from build123d import *

# Parameters (mm, degrees)
F0_R      = 19.05
F1_DEPTH  = 15.875
F2_R      = 9.525
F3_DEPTH  = 12.7
F5_R      = 1.5875
F6_DEPTH  = 25.4
F7_R      = 1.582292
F8_DEPTH  = 25.4
F9_R      = 1.5875
F10_DEPTH = 25.4
F11_R     = 1.5875
F12_DEPTH = 25.4
F13_R     = 1.5875
F14_DEPTH = 25.4
F15_R     = 1.5875
F16_DEPTH = 25.4
F17_R     = 1.5875
F18_DEPTH = 25.4
F19_R     = 1.5875
F20_DEPTH = 25.4
F21_R     = 4.7625
F22_DEPTH = 1.5875
F23_R     = 2.38125
F24_DEPTH = 1.5875
F26_R     = 18.052575
F26_R_2   = 9.68479
F27_DEPTH = 13.462
F28_R     = 3.175
F29_DEPTH = 9.652
F30_R     = 1.5875
F31_DEPTH = 10.668


with BuildPart() as f1:
    # F0 (on Front) → F1 (new body)
    with BuildSketch(Plane.XZ):
        Circle(F0_R)
    extrude(amount=-F1_DEPTH)

    # F2 (on face) → F3 (cut)
    with BuildSketch(Plane.XZ):
        Circle(F2_R)
    extrude(amount=-F3_DEPTH, mode=Mode.SUBTRACT)

    # F5 (on face) → F6 (cut)
    with BuildSketch(Plane.XZ.offset(-12.7)):
        with Locations((0, 7.420709)):
            Circle(F5_R)
    extrude(amount=-F6_DEPTH, mode=Mode.SUBTRACT)

    # F7 (on face) → F8 (cut)
    with BuildSketch(Plane.XZ.offset(-12.7)):
        with Locations((0, -7.351812)):
            Circle(F7_R)
    extrude(amount=-F8_DEPTH, mode=Mode.SUBTRACT)

    # F9 (on face) → F10 (cut)
    with BuildSketch(Plane.XZ.offset(-12.7)):
        with Locations((-7.360636, 0)):
            Circle(F9_R)
    extrude(amount=-F10_DEPTH, mode=Mode.SUBTRACT)

    # F11 (on face) → F12 (cut)
    with BuildSketch(Plane.XZ.offset(-12.7)):
        with Locations((7.366985, 0)):
            Circle(F11_R)
    extrude(amount=-F12_DEPTH, mode=Mode.SUBTRACT)

    # F13 (on face) → F14 (cut)
    with BuildSketch(Plane.XZ.offset(-12.7)):
        with Locations((-5.115572, 5.085843)):
            Circle(F13_R)
    extrude(amount=-F14_DEPTH, mode=Mode.SUBTRACT)

    # F15 (on face) → F16 (cut)
    with BuildSketch(Plane.XZ.offset(-12.7)):
        with Locations((5.301525, 5.085843)):
            Circle(F15_R)
    extrude(amount=-F16_DEPTH, mode=Mode.SUBTRACT)

    # F17 (on face) → F18 (cut)
    with BuildSketch(Plane.XZ.offset(-12.7)):
        with Locations((-5.205374, -5.196551)):
            Circle(F17_R)
    extrude(amount=-F18_DEPTH, mode=Mode.SUBTRACT)

    # F19 (on face) → F20 (cut)
    with BuildSketch(Plane.XZ.offset(-12.7)):
        with Locations((5.166822, -5.016946)):
            Circle(F19_R)
    extrude(amount=-F20_DEPTH, mode=Mode.SUBTRACT)

    # F21 (on face) → F22 (join)
    with BuildSketch(Plane.XZ.offset(-12.7)):
        Circle(F21_R)
    extrude(amount=F22_DEPTH)

    # F23 (on face) → F24 (join)
    with BuildSketch(Plane.XZ.offset(-11.1125)):
        Circle(F23_R)
    extrude(amount=F24_DEPTH)

    # F26 (on face) → F27 (cut)
    with BuildSketch(Plane(origin=(0, 15.875, 0), x_dir=(-1, 0, 0), z_dir=(0, 1, 0))):
        Circle(F26_R)
        Circle(F26_R_2, mode=Mode.SUBTRACT)
    extrude(amount=-F27_DEPTH, mode=Mode.SUBTRACT)

    # F28 (on face) → F29 (join)
    with BuildSketch(Plane(origin=(0, 15.875, 0), x_dir=(-1, 0, 0), z_dir=(0, 1, 0))):
        Circle(F28_R)
    extrude(amount=F29_DEPTH)

    # F30 (on face) → F31 (cut)
    with BuildSketch(Plane(origin=(0, 25.527, 0), x_dir=(-1, 0, 0), z_dir=(0, 1, 0))):
        Circle(F30_R)
    extrude(amount=-F31_DEPTH, mode=Mode.SUBTRACT)


solid = f1.part
The listing builds one solid part. Answer for the finished solid, in the listing's coordinates (mm). A direction names the side the tool comes from. Coordinates: 2 decimals unless noted, no trailing zeros. Loops run counter-clockwise (first coordinate to the right, second up) from the corner with the lowest first, then second, coordinate; pieces in that order, holes last. Notation, with made-up numbers: (62, -17.75) -> (76, -17.75) arc R21 cw to (76, -3.75) -> close; hole circle Ø10 at (56, 55). An arc over 180 degrees is marked (long way). Answer in a Markdown table with one row per item. Add a question column.
1. The part is cut by section A-A, the plane y = 6.75. Write down the section's boundary in (x, z) (3 decimals), then the cut area to 3 significant figures.
2. Consider line 1 (Z direction, x = 0, y = 13.55); line 2 (Z direction, x = 0, y = 10.75) (3 decimals); line 3 (Z direction, x = -1.5, y = 7.5). Determine where each line is inside the solid, lowest interval first. Write a range as [from, to].
3. Determine the mould class of faces 4 (the flat face through (4, 0, 9)), 5 (the flat face through (0, 9.525, 0)), 6 (the cylindrical face through (0.69, 20.63, -3.1)) for opening direction Z: +Z half, -Z half, draft (parallel to the pull), parting line (faces both ways), or undercut.
4. For faces 1 (the flat face through (2, 11.112, -2)), 2 (the cylindrical face through (-5.46, 14.265, 3.536)), 3 (the flat face through (0, 15.875, -4)), determine the directions among +Z, -Z, +X, -X, +Y, -Y from which every point of the face is accessible in a straight line to the end or side of a thin tool.
5. The part is cut by section B-B, the plane z = 0. Count the separate pieces of the cut face and the enclosed holes in it, then the cut area to 3 significant figures.
6. Flat-ended cylindrical pins translate along their axes: P1, Ø6, axis at x = -2, z = -3.5, coming from the -Y side (3 decimals); P2, Ø12, axis at x = 11, y = 3.5, coming from the +Z side; P3, Ø18, axis at x = -6.5, z = -8.5, coming from the +Y side; P4, Ø5, axis at x = 5.17, z = -5.02, coming from the +Y side (3 decimals). Find the tip coordinate at first contact, or state that the pin passes through.
Answer below:
| question | item | result |
|---|---|---|
| 1 | outline | circle Ø38.1 at (0, 0); circle Ø19.37 at (0, 0); hole circle Ø36.105 at (0, 0); hole circle Ø19.05 at (0, 0) |
| 1 | area | 126 mm2 |
| 2 | line 1 | [-19.05, -18.05], [-9.68, -8.93], [-5.77, 5.83], [9.01, 9.68], [18.05, 19.05] |
| 2 | line 2 | [-19.05, -18.053], [-9.685, -9.525], [-2.381, 2.381], [9.525, 9.685], [18.053, 19.05] |
| 2 | line 3 | [-18.99, -17.99], [-9.57, -9.41], [9.41, 9.57], [17.99, 18.99] |
| 3 | face 4 | draft |
| 3 | face 5 | undercut |
| 3 | face 6 | parting line |
| 4 | face 1 | -Y |
| 4 | face 2 | +Y, -Y |
| 4 | face 3 | +Y |
| 5 | separate pieces | 3 |
| 5 | enclosed holes | 0 |
| 5 | area | 168 mm2 |
| 6 | P1 | y = 9.525 |
| 6 | P2 | z = 18.38 |
| 6 | P3 | y = 25.53 |
| 6 | P4 | y = 15.875 |
